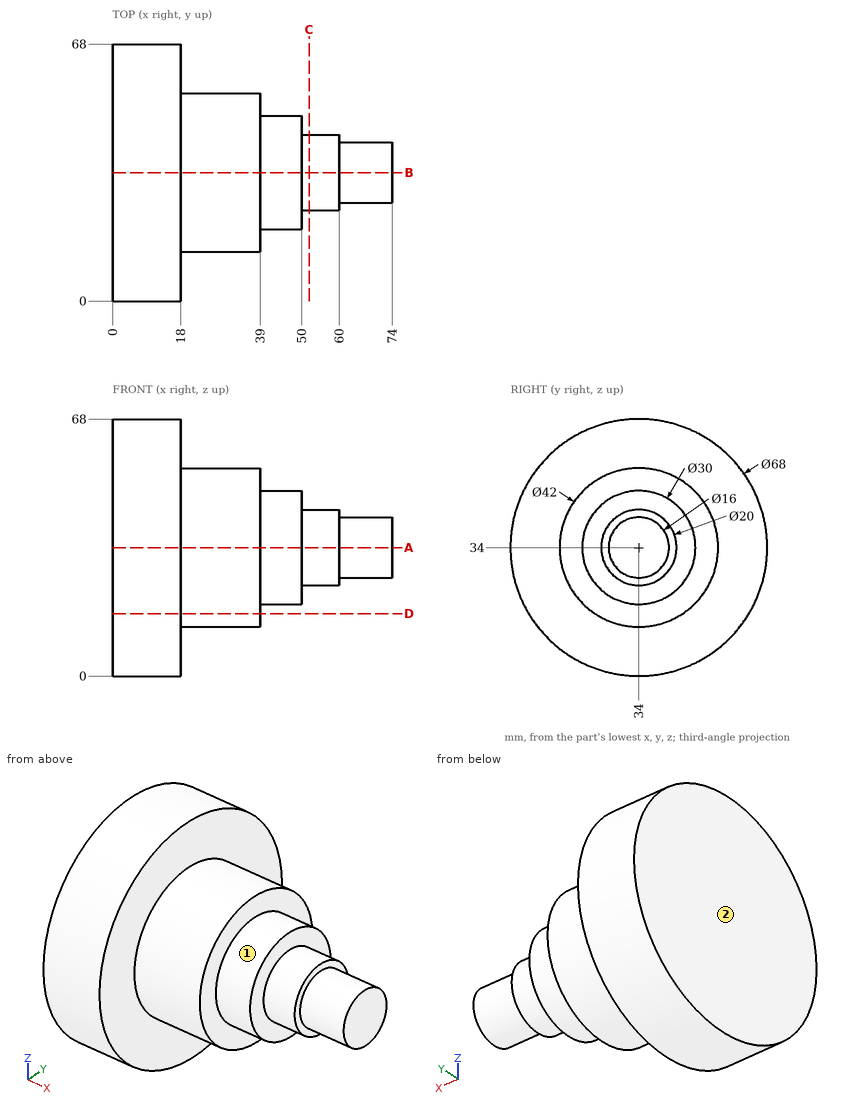
Drawing for the job (mm, zero at the part's lowest x, y, z). A direction names the side the tool comes from. Give positions to 0.01 mm unless a question says otherwise; leave off trailing zeros. Loops run counter-clockwise (first coordinate to the right, second up) from the corner with the lowest first, then second, coordinate; pieces in that order, holes last. Notation, with made-up numbers: (82, 18.25) - (106, 18.25) arc R14 ccw to (106, 35.25) - close; hole circle Ø1 at (-11, -29). An arc over 180 degrees is marked (long way). Write item = value, one per line. Start each with the question number.
1) Drop flat-ended pins along their axis: pin 1 Ø3 at (x, y) = (50.5, 45.5) entering from +Z; pin 2 Ø20.5 at (y, z) = (39, 49) entering from +X; pin 3 Ø6 at (x, y) = (9.5, 50) entering from -Z; pin 4 Ø1 at (x, z) = (9.5, 55.5) entering from +Y. Give the stop position or say it passes through.
2) Band-saw the part on C-C on x = 52. Give the cut face in (y, z), plus the area to 3 significant figures.
3) Probe probe 1 along X at (y, z) = (60, 14.5); probe 2 along X at (y, z) = (47, 23); probe 3 along Z at (x, y) = (4, 33). List the from-to ranges inside material, lowest first. Write a range as from..to.
4) Band-saw the part on A-A on z = 34. Give the cut face in (x, y).
5) Tool access for the marked faces 1 and 2: list every direction of +Z, -Z, +X, -X, +Y, -Y with a clear straight run to the whole face (end or side of a thin tool).
6) Band-saw the part on D-D on z = 16.5. Give the cut face in (x, y), plus the area to 3 significant figures.
Final values:
q1.pin_1 = 45.1
q1.pin_2 = 74
q1.pin_3 = 2.58
q1.pin_4 = 60.74
q2.outline = circle Ø20 at (34, 34)
q2.area = 314 mm²
q3.probe_1 = 0..18
q3.probe_2 = 0..39
q3.probe_3 = 0.01..67.99
q4.outline = (0, 0) - (18, 0) - (18, 13) - (39, 13) - (39, 19) - (50, 19) - (50, 24) - (60, 24) - (60, 26) - (74, 26) - (74, 42) - (60, 42) - (60, 44) - (50, 44) - (50, 49) - (39, 49) - (39, 55) - (18, 55) - (18, 68) - (0, 68) - close
q5.face_1 = +X
q5.face_2 = +Z, -Z, -X, +Y, -Y
q6.outline = (0, 4.85) - (18, 4.85) - (18, 22.39) - (39, 22.39) - (39, 45.61) - (18, 45.61) - (18, 63.15) - (0, 63.15) - close
q6.area = 1,540 mm²
